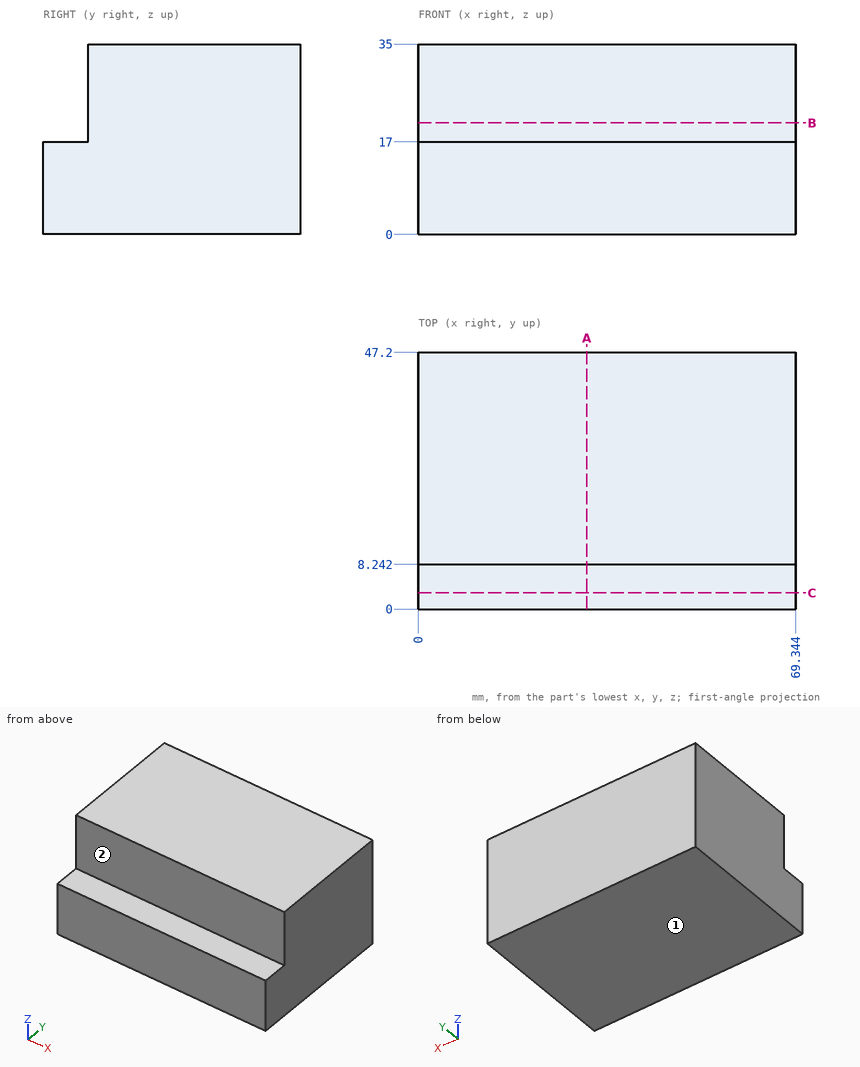
Here's the drawing with two shaded views (mm, measured from the low corner). I have some questions. A direction names the side the tool comes from. Round coordinates to 2 decimals unless told otherwise and drop trailing zeros. Loops run counter-clockwise (first coordinate to the right, second up) from the corner with the lowest first, then second, coordinate; pieces in that order, holes last. Notation, with made-up numbers: M -39,43 L 19,43 A36 ccw 19,79 Z; hole C 74,20.5 d3. An arc over 180 degrees is marked long. Answer as CSV lines item,"result".
1) Imagine slicing it at C-C on y = 3. List the corners of the cut face in (x, z) for me, and give its area (3 significant figures).
From the geometry:
outline,"M 0,0 L 69.34,0 L 69.34,17 L 0,17 Z"
area,"1,180 mm^2"
2) If I drill on probe 1 along Z at (x, y) = (52.5, 6); probe 2 along Y at (x, z) = (38.5, 30), over which ranges is the centre line in solid material (lowest first)?
From the geometry:
probe 1,"0 to 17"
probe 2,"8.24 to 47.2"
3) For pin 1 Ø4 at (x, y) = (40.5, 2.5) entering from +Z, with a flat end and sliding along its axis, tell me the tip position at first contact or that it passes through.
From the geometry:
pin 1,"z = 17"
4) Imagine slicing it at B-B on z = 20.5. List the corners of the cut face in (x, y) for me.
From the geometry:
outline,"M 0,8.24 L 69.34,8.24 L 69.34,47.2 L 0,47.2 Z"
5) Which directions (+Z, -Z, +X, -X, +Y, -Y) give clear straight access to the entire face, cutting with the end or side of a thin tool? Please do the marked faces 1 and 2.
From the geometry:
face 1,"-Z, +X, -X, +Y, -Y"
face 2,"+Z, +X, -X, -Y"
6) Imagine slicing it at A-A on x = 31. List the corners of the cut face in (y, z) for me, and give its area (3 significant figures).
From the geometry:
outline,"M 0,0 L 47.2,0 L 47.2,35 L 8.24,35 L 8.24,17 L 0,17 Z"
area,"1,500 mm^2"
